The listing builds one solid part. Answer for the finished solid, in the listing's coordinates (mm). Face numbers are marked on the shaded views. A direction names the side the tool comes from. Coordinates: 2 decimals unless noted, no trailing zeros. Order: outer loops, then holes, each group sorted by start corner. A loop starts at its lowest first (then second) coordinate and runs counter-clockwise, first axis right, second up. Notation, with made-up numbers: (47, -12) - (70, -12) arc R21 cw to (70, 10) - close; hole circle Ø11 at (80.5, -32.5). An arc over 180 degrees is marked (long way). Use a Markdown table: item, result. Add a question column.
Item 1: The part is cut by section A-A, the plane x = 10.5. Give the vertices of the cut face in (y, z).
Item 2: The part is cut by section C-C, the plane y = 42. Give the vertices of the cut face in (x, z), then the cut area to 3 significant figures.
Item 3: Flat-ended cylindrical pins translate along their axes: P1, Ø3, axis at x = 5, y = 30.5, coming from the +Z side; P2, Ø5, axis at x = 6.5, z = -17.5, coming from the +Y side; P3, Ø0.8, axis at y = 14.5, z = -1, coming from the +X side. Find the tip coordinate at first contact, or state that the pin passes through.
Item 4: For the marked faces 1 and 2, determine the directions among +Z, -Z, +X, -X, +Y, -Y from which every point of the face is accessible in a straight line to the end or side of a thin tool.
Item 5: Find the intervals of material crossed by line 1 along Y through (x, z) = (4.75, -5.25); line 2 along X through (y, z) = (10, -15.75); line 3 along Y through (x, z) = (17.25, -18.5), in increasing order.
Item 6: The part is cut by section B-B, the plane y = 7.5. Give the vertices of the cut face in (x, z).
Item 7: The part is cut by section D-D, the plane y = 31. Give the vertices of the cut face in (x, z).
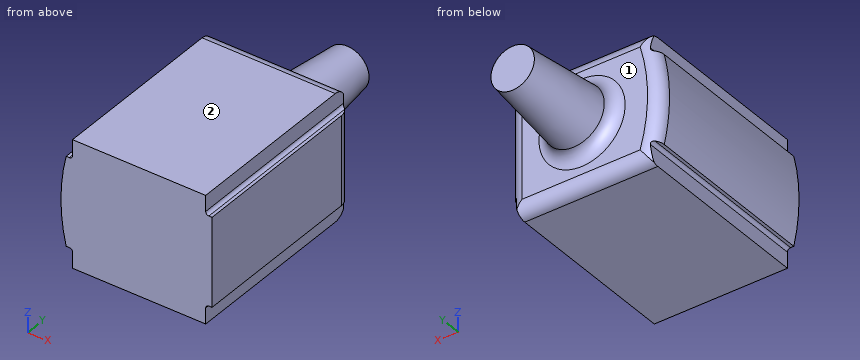
from build123d import *

# Parameters (mm, degrees)
SALIENTE_EXTRUIR1_DEPTH = 30
CROQUIS2_R              = 5
SALIENTE_EXTRUIR2_DEPTH = 15
SALIENTE_EXTRUIR2_TAPER = 6
REDONDEO1_R             = 2
REDONDEO2_R             = 2


with BuildPart() as part:
    # Croquis1 → Saliente-Extruir1 (new body)
    with BuildSketch(Plane(origin=(0, 0, 0), x_dir=(1, 0, 0), z_dir=(0, 1, 0))):
        with BuildLine():
            Line((0, 2.5), (0, 0))
            Line((0, 0), (10.5, 0))
            Line((10.5, 0), (10.5, 20))
            Line((10.5, 20), (0, 20))
            Line((0, 20), (0, 17.5))
            ThreePointArc((0, 17.5), (-0.146446609, 17.146446609), (-0.5, 17))
            Line((-0.5, 17), (-1, 17))
            ThreePointArc((-1, 17), (-1.828095708, 10), (-1, 3))
            Line((-1, 3), (-0.5, 3))
            ThreePointArc((-0.5, 3), (-0.146446609, 2.853553391), (0, 2.5))
        make_face()
        with BuildLine():
            Line((10.5, 20), (10.5, 0))
            Line((10.5, 0), (21, 0))
            Line((21, 0), (21, 2.5))
            ThreePointArc((21, 2.5), (21.146446609, 2.853553391), (21.5, 3))
            Line((21.5, 3), (22, 3))
            Line((22, 3), (22, 17))
            Line((22, 17), (21.5, 17))
            ThreePointArc((21.5, 17), (21.146446609, 17.146446609), (21, 17.5))
            Line((21, 17.5), (21, 20))
            Line((21, 20), (10.5, 20))
        make_face()
    extrude(amount=SALIENTE_EXTRUIR1_DEPTH)

    # Croquis2 → Saliente-Extruir2 (add)
    with BuildSketch(Plane(origin=(0, 30, 0), x_dir=(1, 0, 0), z_dir=(0, 1, 0))):
        with Locations((10.5, 10)):
            Circle(CROQUIS2_R)
    extrude(amount=SALIENTE_EXTRUIR2_DEPTH, taper=SALIENTE_EXTRUIR2_TAPER)

    # Redondeo1
    # the kernel refuses this fillet: 2 mm, written as the material it takes off along each edge
    with BuildSketch(Plane(origin=(26, 30, -20), x_dir=(0, 0, 1), z_dir=(-1, 0, 0)), Plane(origin=(-5, 30, 0), x_dir=(0, 0, -1), z_dir=(1, 0, 0))) as redondeo1_piece_1:
        with BuildLine():
            CenterArc((REDONDEO1_R, -REDONDEO1_R), REDONDEO1_R, 90, 90)
            Line((0, -REDONDEO1_R), (0, 0))
            Line((0, 0), (REDONDEO1_R, 0))
        make_face()
    extrude(amount=31, mode=Mode.SUBTRACT)
    with BuildSketch(Plane(origin=(22, 30, 2), x_dir=(-1, 0, 0), z_dir=(0, 0, -1))) as redondeo1_piece_2:
        with BuildLine():
            CenterArc((REDONDEO1_R, -REDONDEO1_R), REDONDEO1_R, 90, 90)
            Line((0, -REDONDEO1_R), (0, 0))
            Line((0, 0), (REDONDEO1_R, 0))
        make_face()
    extrude(amount=24, mode=Mode.SUBTRACT)
    with BuildSketch(Plane(origin=(28.171904292, 30, -10), x_dir=(-0.92021107903263, 0, -0.391422495553849), z_dir=(0.391422495553849, 0, -0.92021107903263))) as redondeo1_piece_3:
        with BuildLine():
            CenterArc((30 - REDONDEO1_R, -REDONDEO1_R), REDONDEO1_R, 0, 90)
            Line((30 - REDONDEO1_R, 0), (30, 0))
            Line((30, 0), (30, -REDONDEO1_R))
        make_face()
    revolve(axis=Axis((28.171904292, 30, -10), (0, 1, 0)), revolution_arc=46.086080448, mode=Mode.SUBTRACT)

    # Redondeo2
    redondeo2_edges = [part.edges().sort_by_distance(p)[0] for p in [
        (5.5, 30, -10),
    ]]
    fillet(redondeo2_edges, radius=REDONDEO2_R)


solid = part.part
Solution:
| question | item | result |
|---|---|---|
| 1 | outline | (0, -20) - (28, -20) arc R2 ccw to (30, -18) - (30, -16.8) arc R2 cw to (31.79, -14.81) - (45, -13.42) - (45, -6.58) - (31.79, -5.19) arc R2 cw to (30, -3.2) - (30, -2) arc R2 ccw to (28, 0) - (0, 0) - close |
| 2 | outline | circle Ø7.48 at (10.5, -10) |
| 2 | area | 43.9 mm2 |
| 3 | P1 | stops at z = -0.27 |
| 3 | P2 | stops at y = 30.17 |
| 3 | P3 | stops at x = 21 |
| 4 | face 1 | +Y |
| 4 | face 2 | +Z, +X, -X, +Y, -Y |
| 5 | line 1 | y = 0 to 30 |
| 5 | line 2 | x = -1.27 to 22 |
| 5 | line 3 | y = 0 to 29.94 |
| 6 | outline | (-1, -17) - (-0.5, -17) arc R0.5 cw to (0, -17.5) - (0, -20) - (21, -20) - (21, -17.5) arc R0.5 cw to (21.5, -17) - (22, -17) - (22, -3) - (21.5, -3) arc R0.5 cw to (21, -2.5) - (21, 0) - (0, 0) - (0, -2.5) arc R0.5 cw to (-0.5, -3) - (-1, -3) arc R30 ccw to start |
| 7 | outline | circle Ø10.14 at (10.5, -10) |
